```python
from build123d import *

# Parameters (mm, degrees)
DODANIE_WYCI_GNI_CIE1_DEPTH = 6
SZKIC2_R                    = 1.55
WYTNIJ_WYCI_GNI_CIE1_DEPTH  = 6
SZKIC5_R                    = 4.05
WYTNIJ_WYCI_GNI_CIE3_DEPTH  = 6
SZKIC7_R                    = 1.55
WYTNIJ_WYCI_GNI_CIE5_DEPTH  = 10


with BuildPart() as part:
    # Szkic1 → Dodanie-wyciągnięcie1 (new body)
    with BuildSketch(Plane.XY):
        with BuildLine():
            Line((-200.181077779, 116.924844228), (-200.181077779, 76.924846477))
            ThreePointArc((-200.181077779, 76.924846477), (-188.181077779, 64.924846477), (-176.181077779, 76.924846477))
            Line((-176.181077779, 76.924846477), (-176.181077779, 116.924844163))
            ThreePointArc((-176.181077779, 116.924844163), (-188.181077747, 128.924846477), (-200.181077779, 116.924844228))
        make_face()
    extrude(amount=DODANIE_WYCI_GNI_CIE1_DEPTH)

    # Szkic2 → Wytnij-wyciągnięcie1 (cut)
    with BuildSketch(Plane.XY.offset(6)):
        with Locations((-196.181077779, 98.324819795)):
            Circle(SZKIC2_R)
        with Locations((-180.181077779, 98.324819795)):
            Circle(SZKIC2_R)
        with Locations((-188.181077779, 67.924846477)):
            Circle(SZKIC2_R)
    extrude(amount=-WYTNIJ_WYCI_GNI_CIE1_DEPTH, mode=Mode.SUBTRACT)

    # Szkic5 → Wytnij-wyciągnięcie3 (cut)
    with BuildSketch(Plane.XY.offset(6)):
        with Locations((-188.181077779, 116.924846477)):
            Circle(SZKIC5_R)
    extrude(amount=-WYTNIJ_WYCI_GNI_CIE3_DEPTH, mode=Mode.SUBTRACT)

    # Szkic7 → Wytnij-wyciągnięcie5 (cut)
    with BuildSketch(Plane.XY.offset(6)):
        with Locations((-188.181077779, 76.924846477)):
            Circle(SZKIC7_R)
    extrude(amount=-WYTNIJ_WYCI_GNI_CIE5_DEPTH, mode=Mode.SUBTRACT)


solid = part.part
```
Geometry: final body of the model. Coordinates: model frame, mm. Give positions to 0.01 mm unless a question says otherwise; leave off trailing zeros. Loops run counter-clockwise (first coordinate to the right, second up) from the corner with the lowest first, then second, coordinate; pieces in that order, holes last. Notation, with made-up numbers: (-36.75, 32.5) -> (0.25, 32.5) arc R16 ccw to (0.25, 49.5) -> close; hole circle Ø6 at (17, -13.5). An arc over 180 degrees is marked (long way). Return JSON: item names as keys, results as strings.
Item 1: Section C-C, the plane y = 99. Output: boundary loops of the cut face in (x, z), plus the area to 3 significant figures.
Filled in:
{"outline": "(-200.18, 0) -> (-197.58, 0) -> (-197.58, 6) -> (-200.18, 6) -> close; (-194.79, 0) -> (-181.58, 0) -> (-181.58, 6) -> (-194.79, 6) -> close; (-178.79, 0) -> (-176.18, 0) -> (-176.18, 6) -> (-178.79, 6) -> close", "area": "111 mm^2"}
Item 2: Line query: line 1 (Y direction, x = -188, z = 1.95); line 2 (X direction, y = 77, z = 1); line 3 (Y direction, x = -181.5, z = 2.55). Output: solid intervals per line, ascending.
Filled in:
{"line 1": "64.93 to 66.39, 69.46 to 75.39, 78.46 to 112.88, 120.97 to 128.92", "line 2": "-200.18 to -189.73, -186.63 to -176.18", "line 3": "66.96 to 97.51, 99.14 to 126.89"}
Item 3: Section A-A, the plane x = -187.25. Output: boundary loops of the cut face in (y, z).
Filled in:
{"outline": "(64.96, 0) -> (66.69, 0) -> (66.69, 6) -> (64.96, 6) -> close; (69.16, 0) -> (75.69, 0) -> (75.69, 6) -> (69.16, 6) -> close; (78.16, 0) -> (112.98, 0) -> (112.98, 6) -> (78.16, 6) -> close; (120.87, 0) -> (128.89, 0) -> (128.89, 6) -> (120.87, 6) -> close"}
Item 4: Section B-B, the plane y = 77.5. Output: boundary loops of the cut face in (x, z).
Filled in:
{"outline": "(-200.18, 0) -> (-189.62, 0) -> (-189.62, 6) -> (-200.18, 6) -> close; (-186.74, 0) -> (-176.18, 0) -> (-176.18, 6) -> (-186.74, 6) -> close"}
Item 5: Section D-D, the plane z = 2.3. Output: boundary loops of the cut face in (x, y), plus the area to 3 significant figures.
Filled in:
{"outline": "(-200.18, 76.92) arc R12 ccw to (-176.18, 76.92) -> (-176.18, 116.92) arc R12 ccw to (-200.18, 116.92) -> close; hole circle Ø3.1 at (-196.18, 98.32); hole circle Ø8.1 at (-188.18, 116.92); hole circle Ø3.1 at (-188.18, 67.92); hole circle Ø3.1 at (-188.18, 76.92); hole circle Ø3.1 at (-180.18, 98.32)", "area": "1,330 mm^2"}
Item 6: Mould query, pull axis X, two halves, no side actions, for faces 1 (the cylindrical face through (-189.73, 67.99, 3.04)), 2 (the cylindrical face through (-187.917, 128.922, 2.958)), 3 (the flat face through (-188, 97, 6)). Classes: released by +X, released by -X, zero draft, split by the parting line, or undercut.
Filled in:
{"face 1": "undercut", "face 2": "split by the parting line", "face 3": "zero draft"}
Item 7: Pin query (flat end, axial travel): P1, Ø3, axis at x = -181.5, z = 5, coming from the -Y side. Return the tip coordinate at first contact, or that it passes through.
Filled in:
{"P1": "y = 66.1"}
